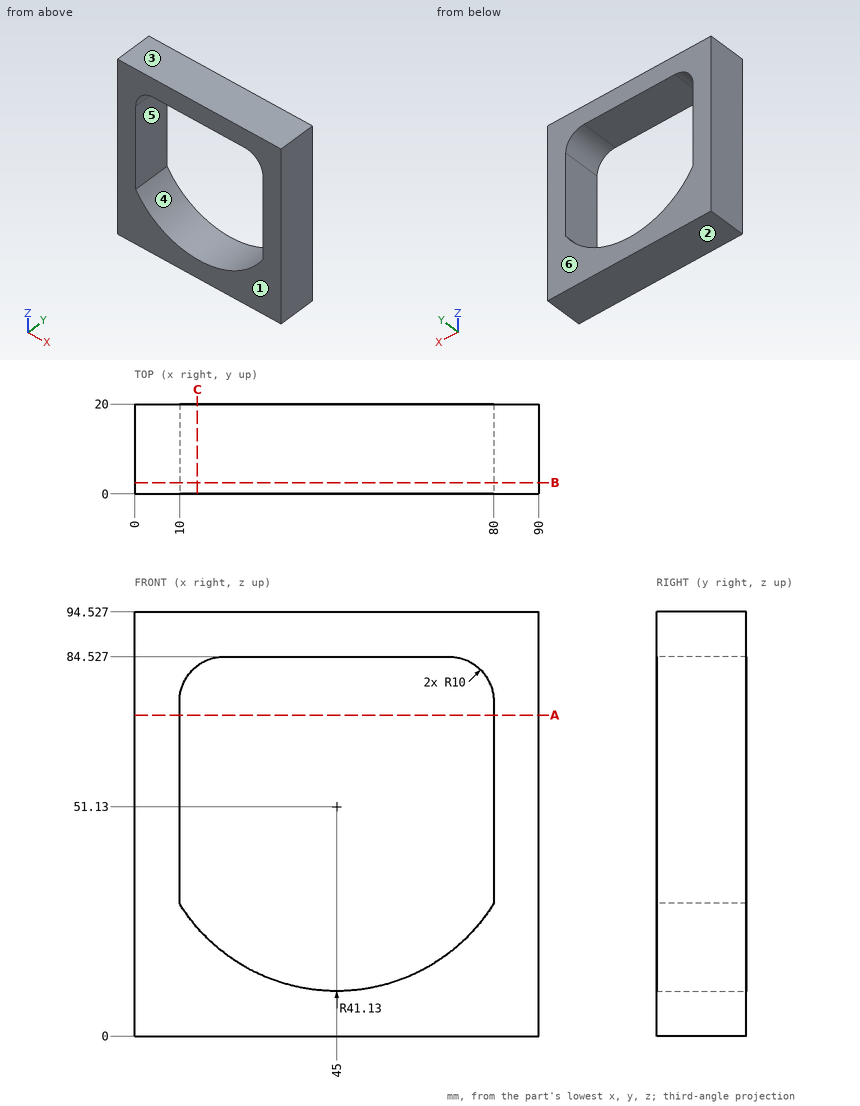
Here's the drawing with two shaded views (mm, measured from the low corner). I have some questions. A direction names the side the tool comes from. Round coordinates to 2 decimals unless told otherwise and drop trailing zeros. Loops run counter-clockwise (first coordinate to the right, second up) from the corner with the lowest first, then second, coordinate; pieces in that order, holes last. Notation, with made-up numbers: (47, 47.5) - (70, 47.5) arc R15 cw to (70, 67.5) - close; hole circle Ø4 at (52, 48.25). An arc over 180 degrees is marked (long way). Use CSV: the item, a comma, the result in double quotes.
Item 1: If we section it at C-C on x = 14: List the corners of the cut face in (y, z) for me.
Here are the results:
outline,"(0, 0) - (20, 0) - (20, 24.1) - (0, 24.1) - close; (0, 82.53) - (20, 82.53) - (20, 94.53) - (0, 94.53) - close"
Item 2: If we mould it in two halves opening along Z, with no side actions, what happens to the marked faces 1, 2, 3 and 4? For each: pulls with the +Z half, pulls with the -Z half, needs draft (parallel to the pull), parting line crosses it, or undercut.
Here are the results:
face 1,"needs draft"
face 2,"pulls with the -Z half"
face 3,"pulls with the +Z half"
face 4,"undercut"
Item 3: I need wall thicknesses on L1, parallel to X at y = 10.5, z = 33; L2, parallel to Z at x = 44.5, y = 12; L3, parallel to X at y = 6.5, z = 17.5. Which ranges of each line are inside material? Lowest first, please. Write a range as [from, to].
Here are the results:
L1,"x = [0, 10], [80, 90]"
L2,"z = [0, 10], [84.53, 94.53]"
L3,"x = [0, 21.32], [68.68, 90]"
Item 4: If we section it at B-B on y = 2.5: List the corners of the cut face in (x, z) for me.
Here are the results:
outline,"(0, 0) - (90, 0) - (90, 94.53) - (0, 94.53) - close; hole (10, 29.53) arc R41.13 ccw to (80, 29.53) - (80, 74.53) arc R10 ccw to (70, 84.53) - (20, 84.53) arc R10 ccw to (10, 74.53) - close"
Item 5: For the marked faces 5 and 6, which set-ups out of +Z, -Z, +X, -X, +Y, -Y let a thin tool reach every point of the face, with its end or its side?
Here are the results:
face 5,"+Y, -Y"
face 6,"+Z, -Z, +X, -X, +Y"
Item 6: Will this pin go through, and if not, where does the flat tip stop? pin 1 (6 mm diameter, centred on x = 48, y = 13.5, fed in from -Z).
Here are the results:
pin 1,"stops at z = 0"
Item 7: If we section it at A-A on z = 71.5: List the corners of the cut face in (x, y) for me, then the cut area to 3 significant figures.
Here are the results:
outline,"(0, 0) - (10, 0) - (10, 20) - (0, 20) - close; (80, 0) - (90, 0) - (90, 20) - (80, 20) - close"
area,"400 mm²"
